from build123d import *

# Parameters (mm, degrees)
F0_W     = 60
F0_H     = 20
F0_R     = 4
F1_DEPTH = 2.4
F2_DEPTH = 25
F3_SIZE  = 2
F4_SIZE  = 1.5


with BuildPart() as f1:
    # F0 (on Top) → F1 (new body)
    with BuildSketch(Plane.XY):
        Rectangle(F0_W, F0_H)
        with Locations((-20, 0)):
            Circle(F0_R, mode=Mode.SUBTRACT)
        with BuildLine():
            ThreePointArc((24, 0), (20, -4), (16, 0))
            ThreePointArc((16, 0), (20, 4), (24, 0))
        make_face(mode=Mode.SUBTRACT)
        with Locations((-20, 0)):
            Circle(F0_R)
        with BuildLine():
            ThreePointArc((24, 0), (20, 4), (16, 0))
            ThreePointArc((16, 0), (20, -4), (24, 0))
        make_face()
    extrude(amount=F1_DEPTH)

    # F0 (on Top) → F2 (join)
    with BuildSketch(Plane.XY):
        with Locations((-20, 0)):
            Circle(F0_R)
        with BuildLine():
            ThreePointArc((24, 0), (20, 4), (16, 0))
            ThreePointArc((16, 0), (20, -4), (24, 0))
        make_face()
    extrude(amount=F2_DEPTH)

    # F3
    f3_edges = [f1.edges().sort_by_distance(p)[0] for p in [
        (0, -10, 0),
        (30, 0, 0),
        (0, 10, 0),
        (-30, 0, 0),
    ]]
    chamfer(f3_edges, length=F3_SIZE)

    # F4
    f4_edges = [f1.edges().sort_by_distance(p)[0] for p in [
        (-24, 0, 25),
        (24, 0, 25),
    ]]
    chamfer(f4_edges, length=F4_SIZE)


solid = f1.part
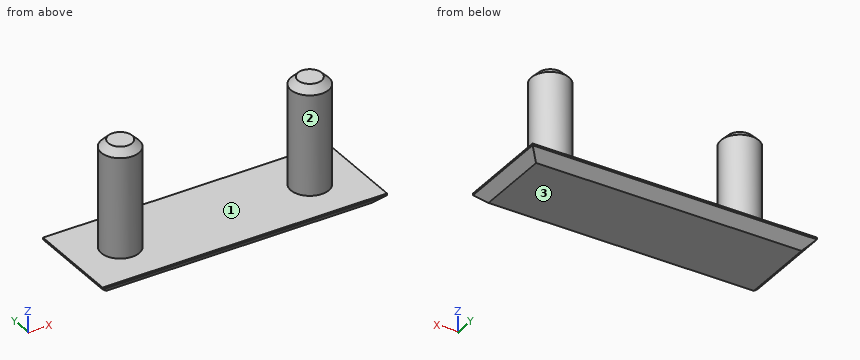
Geometry: final body of the model. Coordinates: model frame, mm. Face numbers are marked on the shaded views. Round coordinates to 2 decimals unless told otherwise and drop trailing zeros. Write each loop counter-clockwise with the first axis right and the second up, starting at its lowest first coordinate (ties: lowest second). Pieces come first, ordered by that corner, then holes. Notation, with made-up numbers: M -29.75,-29.75 L -7.75,-29.75 A28 cw -7.75,-10.75 Z; hole C 20.5,2 d1. An arc over 180 degrees is marked long. Write item = value, one per line.
Item 1: Section query B-B on x = 20. Return loops of the section in (y, z).
Findings:
outline = M -10,2 L -8,0 L 8,0 L 10,2 L 10,2.4 L 4,2.4 L 4,23.5 L 2.5,25 L -2.5,25 L -4,23.5 L -4,2.4 L -10,2.4 Z
Item 2: Section query C-C on z = 5. Return loops of the section in (x, y), then the cut area to 3 significant figures.
Findings:
outline = C -20,0 d8; C 20,0 d8
area = 101 mm^2
Item 3: Pull-direction query (X, two-part tool) for the marked faces 1, 2 and 3; classes: pulls with the +X half, pulls with the -X half, needs draft (parallel to the pull), parting line crosses it, or undercut.
Findings:
face_1 = undercut
face_2 = undercut
face_3 = needs draft
Item 4: Section query A-A on y = -5.75. Return loops of the section in (x, z), then the cut area to 3 significant figures.
Findings:
outline = M -30,2 L -28,0 L 28,0 L 30,2 L 30,2.4 L -30,2.4 Z
area = 140 mm^2
Item 5: Pin query (flat end, axial travel): P1, Ø6, axis at x = 0.5, y = -4, coming from the +Z side; P2, Ø1.5, axis at x = -19, z = 22, coming from the -Y side; P3, Ø1.5, axis at x = 16.5, z = 20.5, coming from the +Y side. Return the tip coordinate at first contact, or that it passes through.
Findings:
P1 = 2.4
P2 = -3.99
P3 = 2.9
Item 6: Section query D-D on y = 0. Return loops of the section in (x, z).
Findings:
outline = M -30,2 L -28,0 L 28,0 L 30,2 L 30,2.4 L 24,2.4 L 24,23.5 L 22.5,25 L 17.5,25 L 16,23.5 L 16,2.4 L -16,2.4 L -16,23.5 L -17.5,25 L -22.5,25 L -24,23.5 L -24,2.4 L -30,2.4 Z
Item 7: Material intervals for line 1 along Z through (x, y) = (-4.5, -4.5); line 2 along X through (y, z) = (-1.25, 7.5); line 3 along X through (y, z) = (0.75, 9.75), sorted ascending. Write a range as [from, to].
Findings:
line_1 = [0, 2.4]
line_2 = [-23.8, -16.2], [16.2, 23.8]
line_3 = [-23.93, -16.07], [16.07, 23.93]
